Could you check a few things on this model? Use its own coordinates, in mm. Face numbers are marked on the shaded views. Round coordinates to 2 decimals unless told otherwise and drop trailing zeros. Write each loop counter-clockwise with the first axis right and the second up, starting at its lowest first coordinate (ties: lowest second). Pieces come first, ordered by that corner, then holes. Notation, with made-up numbers: (5.5, 9.5) -> (11.5, 9.5) arc R29 cw to (11.5, 45.5) -> close; hole circle Ø4 at (57.5, 71.25). An arc over 180 degrees is marked (long way). One line per question, with ' | ' between items. Start each with the question number.
1. For pin 1 Ø8 at (x, y) = (3.5, 1.5) entering from +Z, with a flat end and sliding along its axis, tell me the tip position at first contact or that it passes through.
2. Imagine slicing it at B-B, the plane z = 13.5. List the corners of the cut face in (x, y) for me, and give its area (3 significant figures).
3. If I drill on line 1 along X through (y, z) = (-3.5, 19.25); line 2 along Y through (x, z) = (-7.5, 17.25); line 3 along Z through (x, y) = (-6.25, -1.5), over which ranges is the centre line in solid material (lowest first)? Write a range as [from, to].
4. Imagine slicing it at A-A, the plane x = 2. List the corners of the cut face in (y, z) for me.
5. Thinking about a two-plate mould opening in X: for the marked faces 1, 2, 3 and 4, which applies, released by +X, released by -X, zero draft, split by the parting line, or undercut?
6. Imagine slicing it at C-C, the plane y = 4. List the corners of the cut face in (x, z) for me.
from build123d import *

# Parameters (mm, degrees)
SKETCH2_W           = 22
SKETCH2_H           = 20
SKETCH2_W_2         = 20
SKETCH2_H_2         = 18
BOSS_EXTRUDE1_DEPTH = 10
SKETCH2_2_W         = 20
SKETCH2_2_H         = 18
BOSS_EXTRUDE2_DEPTH = 1
SKETCH2_3_W         = 22
SKETCH2_3_H         = 20
SKETCH2_3_W_2       = 20
SKETCH2_3_H_2       = 18
BOSS_EXTRUDE3_DEPTH = 1
SKETCH2_4_W         = 22
SKETCH2_4_H         = 20
SKETCH2_4_W_2       = 20
SKETCH2_4_H_2       = 18
BOSS_EXTRUDE4_DEPTH = 26


with BuildPart() as part:
    # Sketch2 → Boss-Extrude1 (new body)
    with BuildSketch(Plane.XY):
        Rectangle(SKETCH2_W, SKETCH2_H)
        Rectangle(SKETCH2_W_2, SKETCH2_H_2, mode=Mode.SUBTRACT)
    extrude(amount=BOSS_EXTRUDE1_DEPTH)



with BuildPart() as body_2:
    # Sketch2<2> → Boss-Extrude2 (new body)
    with BuildSketch(Plane.XY):
        Rectangle(SKETCH2_2_W, SKETCH2_2_H)
    extrude(amount=-BOSS_EXTRUDE2_DEPTH)


with BuildPart() as part_1:
    add(part.part)

    add(body_2.part)  # Boss-Extrude3 merges body 2
    # Sketch2<3> → Boss-Extrude3 (add)
    with BuildSketch(Plane.XY):
        Rectangle(SKETCH2_3_W, SKETCH2_3_H)
        Rectangle(SKETCH2_3_W_2, SKETCH2_3_H_2, mode=Mode.SUBTRACT)
    extrude(amount=-BOSS_EXTRUDE3_DEPTH)

    # Sketch2<4> → Boss-Extrude4 (add)
    with BuildSketch(Plane.XY):
        Rectangle(SKETCH2_4_W, SKETCH2_4_H)
        Rectangle(SKETCH2_4_W_2, SKETCH2_4_H_2, mode=Mode.SUBTRACT)
    extrude(amount=BOSS_EXTRUDE4_DEPTH)


solid = part_1.part
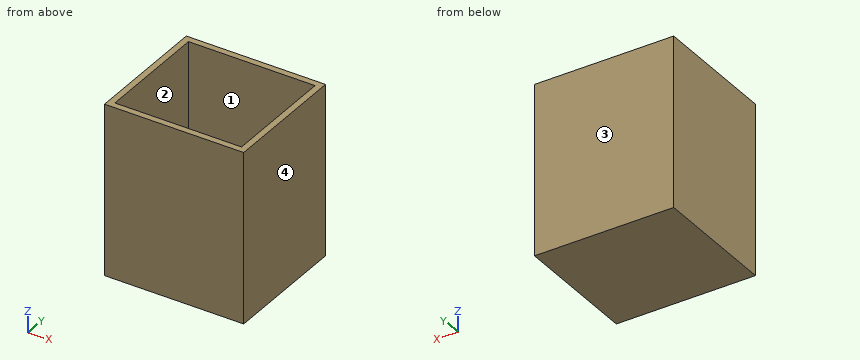
Geometry results:
1) pin 1: stops at z = 0
2) outline: (-11, -10) -> (11, -10) -> (11, 10) -> (-11, 10) -> close; hole (-10, -9) -> (10, -9) -> (10, 9) -> (-10, 9) -> close | area: 80.0 mm2
3) line 1: x = [-11, -10], [10, 11] | line 2: y = [-10, -9], [9, 10] | line 3: z = [-1, 0]
4) outline: (-10, -1) -> (10, -1) -> (10, 26) -> (9, 26) -> (9, 0) -> (-9, 0) -> (-9, 26) -> (-10, 26) -> close
5) face 1: undercut | face 2: undercut | face 3: zero draft | face 4: released by +X
6) outline: (-11, -1) -> (11, -1) -> (11, 26) -> (10, 26) -> (10, 0) -> (-10, 0) -> (-10, 26) -> (-11, 26) -> close
